```python
from build123d import *

# Parameters (mm, degrees)
F0_R     = 7.5
F1_DEPTH = 12
F2_R     = 1
F3_W     = 1
F3_H     = 1


# Not quite as in the source:
# - a pattern or mirror of a feature is missing from the dataset's text; its kind, count and spacing are read off the source's solid


with BuildPart() as f1:
    # F0 (on Front) → F1 (new body, symmetric)
    with BuildSketch(Plane.XZ):
        Circle(F0_R)
        with BuildLine():
            ThreePointArc((3.0970921684, 2.5314067434), (3.69551813, 1.5307337295), (3.9799497484, 0.4))
            Line((3.9799497484, 0.4), (6.2799497484, 0.4))
            Line((6.2799497484, 0.4), (6.2799497484, -0.4))
            Line((6.2799497484, -0.4), (3.9799497484, -0.4))
            ThreePointArc((3.9799497484, -0.4), (3.69551813, -1.5307337295), (3.0970921684, -2.5314067434))
            Line((3.0970921684, -2.5314067434), (4.7234377651, -4.1577523401))
            Line((4.7234377651, -4.1577523401), (4.1577523401, -4.7234377651))
            Line((4.1577523401, -4.7234377651), (2.5314067434, -3.0970921684))
            ThreePointArc((2.5314067434, -3.0970921684), (1.5307337295, -3.69551813), (0.4, -3.9799497484))
            Line((0.4, -3.9799497484), (0.4, -6.2799497484))
            Line((0.4, -6.2799497484), (-0.4, -6.2799497484))
            Line((-0.4, -6.2799497484), (-0.4, -3.9799497484))
            ThreePointArc((-0.4, -3.9799497484), (-1.5307337295, -3.69551813), (-2.5314067434, -3.0970921684))
            Line((-2.5314067434, -3.0970921684), (-4.1577523401, -4.7234377651))
            Line((-4.1577523401, -4.7234377651), (-4.7234377651, -4.1577523401))
            Line((-4.7234377651, -4.1577523401), (-3.0970921684, -2.5314067434))
            ThreePointArc((-3.0970921684, -2.5314067434), (-3.69551813, -1.5307337295), (-3.9799497484, -0.4))
            Line((-3.9799497484, -0.4), (-6.2799497484, -0.4))
            Line((-6.2799497484, -0.4), (-6.2799497484, 0.4))
            Line((-6.2799497484, 0.4), (-3.9799497484, 0.4))
            ThreePointArc((-3.9799497484, 0.4), (-3.69551813, 1.5307337295), (-3.0970921684, 2.5314067434))
            Line((-3.0970921684, 2.5314067434), (-4.7234377651, 4.1577523401))
            Line((-4.7234377651, 4.1577523401), (-4.1577523401, 4.7234377651))
            Line((-4.1577523401, 4.7234377651), (-2.5314067434, 3.0970921684))
            ThreePointArc((-2.5314067434, 3.0970921684), (-1.5307337295, 3.69551813), (-0.4, 3.9799497484))
            Line((-0.4, 3.9799497484), (-0.4, 6.2799497484))
            Line((-0.4, 6.2799497484), (0.4, 6.2799497484))
            Line((0.4, 6.2799497484), (0.4, 3.9799497484))
            ThreePointArc((0.4, 3.9799497484), (1.5307337295, 3.69551813), (2.5314067434, 3.0970921684))
            Line((2.5314067434, 3.0970921684), (4.1577523401, 4.7234377651))
            Line((4.1577523401, 4.7234377651), (4.7234377651, 4.1577523401))
            Line((4.7234377651, 4.1577523401), (3.0970921684, 2.5314067434))
        make_face(mode=Mode.SUBTRACT)
    extrude(amount=F1_DEPTH, both=True)

    # F2
    f2_edges = [f1.edges().sort_by_distance(p)[0] for p in [
        (-7.5, -12, 0),
        (-1.530734, -12, 3.695518),
        (-3.695518, -12, 1.530734),
        (-3.695518, -12, -1.530734),
        (-1.530734, -12, -3.695518),
        (1.530734, -12, -3.695518),
        (3.695518, -12, -1.530734),
        (3.695518, -12, 1.530734),
        (1.530734, -12, 3.695518),
        (-7.5, 12, 0),
        (3.695518, 12, -1.530734),
        (3.695518, 12, 1.530734),
        (1.530734, 12, 3.695518),
        (-1.530734, 12, 3.695518),
        (-3.695518, 12, 1.530734),
        (-3.695518, 12, -1.530734),
        (-1.530734, 12, -3.695518),
        (1.530734, 12, -3.695518),
    ]]
    fillet(f2_edges, radius=F2_R)

    # F3 (on Right) → F4 (revolve, cut)
    with BuildSketch(Plane.YZ):
        with Locations((-8, 7)):
            Rectangle(F3_W, F3_H)
    f4 = revolve(axis=Axis((0, 11.2657039426, 0), (0, 1, 0)), mode=Mode.SUBTRACT)

    # F4_copies: F4 across plane
    add(f4.mirror(Plane.ZX), mode=Mode.SUBTRACT)


solid = f1.part
```
Build history of the part. All positions in model axes, mm. A direction names the side the tool comes from. Coordinates: 2 decimals unless noted, no trailing zeros. Write each loop counter-clockwise with the first axis right and the second up, starting at its lowest first coordinate (ties: lowest second). Pieces come first, ordered by that corner, then holes.
1. Drill centre lines: probe 1 along Y at (x, z) = (3, 6.25); probe 2 along X at (y, z) = (-3, 3.25); probe 3 along X at (y, z) = (2.25, 3.5). Where is each one in solid material? Low to high.
Answer block:
probe 1: y = -11.9 to -8.5, -7.5 to 7.5, 8.5 to 11.9
probe 2: x = -6.76 to -3.82, -2.68 to -2.33, 2.33 to 2.68, 3.82 to 6.76
probe 3: x = -6.63 to -4.07, -2.93 to -1.94, 1.94 to 2.93, 4.07 to 6.63
2. Drop flat-ended pins along their axis: pin 1 (5 mm diameter, centred on x = -5.5, y = -5, fed in from -Z); pin 2 (2.5 mm diameter, centred on x = 5, y = -4.5, fed in from -Z); pin 3 (0.7 mm diameter, centred on y = -3, z = 5.5, fed in from -X). Give the stop position or say it passes through.
Answer block:
pin 1: stops at z = -6.87
pin 2: stops at z = -6.5
pin 3: stops at x = -5.45
3. Band-saw the part on A-A, the plane x = 0. Give the cut face in (y, z), and give its area (3 significant figures).
Answer block:
outline: (-12, -6.5) arc R1 ccw to (-11, -7.5) - (-8.5, -7.5) - (-8.5, -6.5) - (-7.5, -6.5) - (-7.5, -7.5) - (7.5, -7.5) - (7.5, -6.5) - (8.5, -6.5) - (8.5, -7.5) - (11, -7.5) arc R1 ccw to (12, -6.5) - (12, -6.28) - (-12, -6.28) - close; (-12, 6.28) - (12, 6.28) - (12, 6.5) arc R1 ccw to (11, 7.5) - (8.5, 7.5) - (8.5, 6.5) - (7.5, 6.5) - (7.5, 7.5) - (-7.5, 7.5) - (-7.5, 6.5) - (-8.5, 6.5) - (-8.5, 7.5) - (-11, 7.5) arc R1 ccw to (-12, 6.5) - close
area: 53.7 mm2
4. Band-saw the part on C-C, the plane z = 0. Give the cut face in (x, y).
Answer block:
outline: (-7.5, -11) arc R1 ccw to (-6.5, -12) - (-6.28, -12) - (-6.28, 12) - (-6.5, 12) arc R1 ccw to (-7.5, 11) - (-7.5, 8.5) - (-6.5, 8.5) - (-6.5, 7.5) - (-7.5, 7.5) - (-7.5, -7.5) - (-6.5, -7.5) - (-6.5, -8.5) - (-7.5, -8.5) - close; (6.28, -12) - (6.5, -12) arc R1 ccw to (7.5, -11) - (7.5, -8.5) - (6.5, -8.5) - (6.5, -7.5) - (7.5, -7.5) - (7.5, 7.5) - (6.5, 7.5) - (6.5, 8.5) - (7.5, 8.5) - (7.5, 11) arc R1 ccw to (6.5, 12) - (6.28, 12) - close
5. 3-axis set-ups, long thin cutter, end or side, ignore diameter. For faces 5 (the cylindrical face through (1.546, -0.154, -3.689)), 6 (the flat face through (3, 7.5, 6)), 7 (the flat face through (-2, 12, 5)): which of +Z, -Z, +X, -X, +Y, -Y reach the whole face in a straight line?
Answer block:
face 5: +Y, -Y
face 6: none
face 7: +Z, -Z, +X, -X, +Y
6. Pull direction Z, two halves, no side cores. Call faces 1 (the cylindrical face through (-3.955, -7.993, -5.158)), 2 (the flat face through (-3.922, -0.168, -3.356)), 3 (the flat face through (-2, -12, 5)), 4 (the flat face through (0.4, 0, -5)): released by +Z, released by -Z, zero draft, split by the parting line, or undercut.
Answer block:
face 1: split by the parting line
face 2: undercut
face 3: zero draft
face 4: undercut
